from build123d import *

# Parameters (mm, degrees)
BOSS_EXTRU_1_DEPTH                                  = 40
ESQUISSE1_4_W                                       = 16
ESQUISSE1_4_H                                       = 96
BOSS_EXTRUDE1_DEPTH                                 = 30
ESQUISSE3_R                                         = 14
ENL_V_MAT_EXTRU_2_DEPTH                             = 40
CONG_1_R                                            = 6
CBORE_FOR_M8_HEX_SOCKET_HEAD_CAP_SCREW2_D           = 9
CBORE_FOR_M8_HEX_SOCKET_HEAD_CAP_SCREW2_CBORE_D     = 15
CBORE_FOR_M8_HEX_SOCKET_HEAD_CAP_SCREW2_CBORE_DEPTH = 8.6
SKETCH7_R                                           = 24.5
CUT_EXTRUDE2_DEPTH                                  = 9
M5_TAPPED_HOLE2_D                                   = 4.2
M5_TAPPED_HOLE2_DEPTH                               = 14
M5_TAPPED_HOLE2_TIP                                 = 1.2618073
SKETCH12_R                                          = 9
CUT_EXTRUDE3_DEPTH                                  = 151
TAP_DRILL_FOR_M6_TAP2_AT_2_COUNT                    = 2
TAP_DRILL_FOR_M6_TAP2_AT_2_PITCH                    = 24
TAP_DRILL_FOR_M6_TAP2_AT_3_COUNT                    = 2
TAP_DRILL_FOR_M6_TAP2_AT_3_PITCH                    = 110
TAP_DRILL_FOR_M6_TAP2_AT_4_COUNT                    = 2
TAP_DRILL_FOR_M6_TAP2_AT_4_PITCH                    = 112.58774356
FILLET2_R                                           = 5
FILLET3_R                                           = 6
FILLET4_R                                           = 2
TAP_DRILL_FOR_M6_TAP1_D                             = 5
TAP_DRILL_FOR_M6_TAP1_DEPTH                         = 23
TAP_DRILL_FOR_M6_TAP1_TIP                           = 1.502151548
FILLET1_R                                           = 1
CHAMFER1_SIZE                                       = 0.5


with BuildPart() as part:
    # Esquisse1 → Boss.-Extru.1 (new body)
    with BuildSketch(Plane.XY):
        Polygon((58.5, -48), (42.5, -48), (42.5, 48), (58.5, 48), (58.5, 105), (-58.5, 105), (-58.5, 48), (-42.5, 48), (-42.5, -48), (-58.5, -48), (-58.5, -85), (-10, -85), (-10, 55), (10, 55), (10, -85), (58.5, -85), align=None)
    extrude(amount=BOSS_EXTRU_1_DEPTH)

    # Esquisse1_4 → Boss-Extrude1 (add)
    with BuildSketch(Plane.XY):
        with Locations((-50.5, 0)):
            Rectangle(ESQUISSE1_4_W, ESQUISSE1_4_H)
        with Locations((50.5, 0)):
            Rectangle(ESQUISSE1_4_W, ESQUISSE1_4_H)
    extrude(amount=BOSS_EXTRUDE1_DEPTH)

    # Esquisse3 → Enl_v. mat.-Extru.2 (cut)
    with BuildSketch(Plane(origin=(0, 105, 0), x_dir=(1, 0, 0), z_dir=(0, 1, 0))):
        with Locations((0, -20)):
            Circle(ESQUISSE3_R)
    extrude(amount=-ENL_V_MAT_EXTRU_2_DEPTH, mode=Mode.SUBTRACT)

    # Cong_1
    cong_1_edges = [part.edges().sort_by_distance(p)[0] for p in [
        (10, 55, 20),
        (-10, 55, 20),
    ]]
    fillet(cong_1_edges, radius=CONG_1_R)

    # CBORE for M8 Hex Socket Head Cap Screw2 (through all)
    with Locations(Plane.XY.offset(40)):
        with Locations((-22.5, 73.5), (22.5, 73.5), (22.5, 16.5), (-22.5, 16.5), (-22.5, -16.5), (22.5, -16.5), (22.5, -73.5), (-22.5, -73.5)):
            CounterBoreHole(CBORE_FOR_M8_HEX_SOCKET_HEAD_CAP_SCREW2_D / 2, CBORE_FOR_M8_HEX_SOCKET_HEAD_CAP_SCREW2_CBORE_D / 2, CBORE_FOR_M8_HEX_SOCKET_HEAD_CAP_SCREW2_CBORE_DEPTH)

    # Sketch7 → Cut-Extrude2 (cut)
    with BuildSketch(Plane(origin=(0, 105, 0), x_dir=(1, 0, 0), z_dir=(0, 1, 0))):
        with Locations((0, -20)):
            Circle(SKETCH7_R)
    extrude(amount=-CUT_EXTRUDE2_DEPTH, mode=Mode.SUBTRACT)

    # M5 Tapped Hole2
    with Locations(Plane(origin=(0, 96, 0), x_dir=(1, 0, 0), z_dir=(0, 1, 0))):
        with Locations((-13.435028843, -6.564971157), (-19, -20), (13.435028843, -6.564971157), (19, -20), (13.435028843, -33.435028843), (-13.435028843, -33.435028843)):
            Hole(M5_TAPPED_HOLE2_D / 2, depth=M5_TAPPED_HOLE2_DEPTH)
            with Locations((0, 0, -(M5_TAPPED_HOLE2_DEPTH + M5_TAPPED_HOLE2_TIP / 2))):  # 118° drill point
                Cone(0, M5_TAPPED_HOLE2_D / 2, M5_TAPPED_HOLE2_TIP, mode=Mode.SUBTRACT)

    # Sketch12 → Cut-Extrude3 (cut, through all)
    with BuildSketch(Plane(origin=(0, 65, 0), x_dir=(1, 0, 0), z_dir=(0, 1, 0))):
        with Locations((0, -20)):
            Circle(SKETCH12_R)
    extrude(amount=-CUT_EXTRUDE3_DEPTH, mode=Mode.SUBTRACT)

    # Sketch14 → Tap Drill for M6 Tap2 (revolve, cut)
    with BuildSketch(Plane(origin=(58.5, 55, 8), x_dir=(0, 0, -1), z_dir=(0, 1, 0))):
        Polygon((0, 0), (0, 11.502151548), (2.5, 10), (2.5, 0), align=None)
    tap_drill_for_m6_tap2 = revolve(axis=Axis((64.85, 55, 8), (-1, 0, 0)), mode=Mode.SUBTRACT)

    # Tap Drill for M6 Tap2 at 2: Tap Drill for M6 Tap2 ×2
    with Locations(*[(0, 0, i * TAP_DRILL_FOR_M6_TAP2_AT_2_PITCH) for i in range(1, TAP_DRILL_FOR_M6_TAP2_AT_2_COUNT)]):
        add(tap_drill_for_m6_tap2, mode=Mode.SUBTRACT)

    # Tap Drill for M6 Tap2 at 3: Tap Drill for M6 Tap2 ×2
    with Locations(*[(0, -i * TAP_DRILL_FOR_M6_TAP2_AT_3_PITCH, 0) for i in range(1, TAP_DRILL_FOR_M6_TAP2_AT_3_COUNT)]):
        add(tap_drill_for_m6_tap2, mode=Mode.SUBTRACT)

    # Tap Drill for M6 Tap2 at 4: Tap Drill for M6 Tap2 ×2
    with Locations(*[Vector(0, -0.977015761, 0.213167075) * (i * TAP_DRILL_FOR_M6_TAP2_AT_4_PITCH) for i in range(1, TAP_DRILL_FOR_M6_TAP2_AT_4_COUNT)]):
        add(tap_drill_for_m6_tap2, mode=Mode.SUBTRACT)

    # Mirror1: Tap Drill for M6 Tap2 across plane
    add(tap_drill_for_m6_tap2.mirror(Plane(origin=(0, 0, 0), x_dir=(0, 0, 1), z_dir=(1, 0, 0))), mode=Mode.SUBTRACT)

    # Mirror1 copy 1 sketch → Mirror1 copy 1 (revolve, cut)
    with BuildSketch(Plane(origin=(-58.5, 55, 32), x_dir=(0, 0, -1), z_dir=(0, 1, 0))):
        Polygon((0, 0), (0, -11.502151548), (2.5, -10), (2.5, 0), align=None)
    revolve(axis=Axis((-64.85, 55, 32), (-1, 0, 0)), mode=Mode.SUBTRACT)

    # Mirror1 copy 2 sketch → Mirror1 copy 2 (revolve, cut)
    with BuildSketch(Plane(origin=(-58.5, -55, 8), x_dir=(0, 0, -1), z_dir=(0, 1, 0))):
        Polygon((0, 0), (0, -11.502151548), (2.5, -10), (2.5, 0), align=None)
    revolve(axis=Axis((-64.85, -55, 8), (-1, 0, 0)), mode=Mode.SUBTRACT)

    # Mirror1 copy 3 sketch → Mirror1 copy 3 (revolve, cut)
    with BuildSketch(Plane(origin=(-58.5, -55, 32), x_dir=(0, 0, -1), z_dir=(0, 1, 0))):
        Polygon((0, 0), (0, -11.502151548), (2.5, -10), (2.5, 0), align=None)
    revolve(axis=Axis((-64.85, -55, 32), (-1, 0, 0)), mode=Mode.SUBTRACT)

    # Fillet2
    fillet2_edges = [part.edges().sort_by_distance(p)[0] for p in [
        (10, -85, 20),
        (-10, -85, 20),
    ]]
    fillet(fillet2_edges, radius=FILLET2_R)

    # Fillet3
    fillet3_edges = [part.edges().sort_by_distance(p)[0] for p in [
        (-42.5, -48, 35),
        (-42.5, 48, 35),
        (42.5, 48, 35),
        (42.5, -48, 35),
    ]]
    fillet(fillet3_edges, radius=FILLET3_R)

    # Fillet4
    fillet4_edges = [part.edges().sort_by_distance(p)[0] for p in [
        (58.5, -48, 35),
        (-58.5, -48, 35),
        (-58.5, 48, 35),
        (58.5, 48, 35),
    ]]
    fillet(fillet4_edges, radius=FILLET4_R)

    # Tap Drill for M6 Tap1
    with Locations(Plane(origin=(0, 105, 0), x_dir=(1, 0, 0), z_dir=(0, 1, 0))):
        with Locations((-51, -30), (-51, -10), (51, -10), (51, -30)):
            Hole(TAP_DRILL_FOR_M6_TAP1_D / 2, depth=TAP_DRILL_FOR_M6_TAP1_DEPTH)
            with Locations((0, 0, -(TAP_DRILL_FOR_M6_TAP1_DEPTH + TAP_DRILL_FOR_M6_TAP1_TIP / 2))):  # 118° drill point
                Cone(0, TAP_DRILL_FOR_M6_TAP1_D / 2, TAP_DRILL_FOR_M6_TAP1_TIP, mode=Mode.SUBTRACT)

    # Fillet1
    fillet1_edges = [part.edges().sort_by_distance(p)[0] for p in [
        (-14.150971698, 100.5, 0),
        (14.150971698, 100.5, 0),
        (14.150971698, 100.5, 40),
        (-14.150971698, 100.5, 40),
    ]]
    fillet(fillet1_edges, radius=FILLET1_R)

    # Chamfer1
    chamfer1_edges = [part.edges().sort_by_distance(p)[0] for p in [
        (15, -73.5, 40),
        (15, -16.5, 40),
        (-30, -16.5, 40),
        (-30, 16.5, 40),
        (15, 16.5, 40),
        (15, 73.5, 40),
        (-30, 73.5, 40),
        (-14, 96, 20),
        (37.753675676, 105, 40),
        (37.753675676, 105, 0),
        (10, -15.5, 40),
        (-36.75, -85, 40),
        (-10, -15.5, 40),
        (-11.464466094, -83.535533906, 40),
        (11.464466094, -83.535533906, 40),
        (-42.5, 0, 40),
        (42.5, 0, 40),
        (-44.257359313, 46.242640687, 40),
        (-44.257359313, -46.242640687, 40),
        (44.257359313, -46.242640687, 40),
        (44.257359313, 46.242640687, 40),
        (52.5, -48, 40),
        (58.5, 77.5, 40),
        (52.5, 48, 40),
        (-58.5, 77.5, 40),
        (-52.5, 48, 40),
        (-52.5, -48, 40),
        (-57.914213562, 48.585786438, 40),
        (-57.914213562, -48.585786438, 40),
        (57.914213562, 48.585786438, 40),
        (57.914213562, -48.585786438, 40),
        (-58.5, 105, 20),
        (58.5, 105, 20),
        (53.5, 105, 30),
        (53.5, 105, 10),
        (-48.5, 105, 10),
        (-48.5, 105, 30),
        (24.5, 105, 20),
        (16.073248028, 105, 0.642997226),
        (16.073248028, 105, 39.357002774),
        (-37.753675676, 105, 40),
        (-24.5, 105, 20),
        (-37.753675676, 105, 0),
        (-16.073248028, 105, 0.642997226),
        (-16.073248028, 105, 39.357002774),
        (-58.5, -67.5, 40),
        (36.75, -85, 40),
        (58.5, -67.5, 40),
        (0, 55, 40),
        (8.242640687, 53.242640687, 40),
        (-8.242640687, 53.242640687, 40),
        (-30, -73.5, 40),
    ]]
    chamfer(chamfer1_edges, length=CHAMFER1_SIZE)


solid = part.part
Source: CAD feature listing. Evaluate the final solid. Frame: model axes, mm. A direction names the side the tool comes from. Coordinates: 2 decimals unless noted, no trailing zeros. Order: outer loops, then holes, each group sorted by start corner. A loop starts at its lowest first (then second) coordinate and runs counter-clockwise, first axis right, second up.
Item 1: Cut plane B-B (y = 1.5). Return loops of the section in (x, z), plus the area to 3 significant figures.
Output values:
outline: (-58.5, 0) - (-10, 0) - (-10, 39.5) - (-10.5, 40) - (-42, 40) - (-42.5, 39.5) - (-42.5, 30) - (-58.5, 30) - close; (10, 0) - (58.5, 0) - (58.5, 30) - (42.5, 30) - (42.5, 39.5) - (42, 40) - (10.5, 40) - (10, 39.5) - close
area: 3,560 mm2
Item 2: Pull-direction query (Z, two-part tool) for faces 6 (the face through (-52.34, 93.09, 27.89)), 7 (the face through (-53.57, 57.44, 8.54)), 8 (the face through (10, -15, 19)), 9 (the face through (26, -20, 31.4)); classes: pulls with the +Z half, pulls with the -Z half, needs draft (parallel to the pull), parting line crosses it, or undercut.
Output values:
face 6: undercut
face 7: undercut
face 8: needs draft
face 9: pulls with the +Z half
Item 3: Cut plane A-A (y = -73.5). Count the separate pieces of the cut face and the enclosed holes in it, plus the area to 3 significant figures.
Output values:
separate pieces: 4
enclosed holes: 0
area: 3,060 mm2
Item 4: First-contact query: P1, Ø12, axis at x = -7, y = 8.5, coming from the +Z side; P2, Ø7.5, axis at x = -22.5, y = -14.5, coming from the +Z side; P3, Ø3, axis at y = 17, z = 36.5, coming from the -X side; P4, Ø5.5, axis at x = 22.5, y = -16.5, coming from the -Z side. Flat tips, straight axial feed; report the tip coordinate or a pass-through.
Output values:
P1: stops at z = 40
P2: stops at z = 31.4
P3: stops at x = -42.5
P4: passes through
Item 5: Set-up query: faces 1 (the face through (44.21, -46.39, 39.64)), 2 (the face through (9.41, 51.595, 20.026)), 3 (the face through (16.548, 68.936, 35.507)), 4 (the face through (-14.4, 88.9, 35.3)), 5 (the face through (53.57, -52.56, 8.54)). Return all of +Z, -Z, +X, -X, +Y, -Y with unobstructed straight access to the full face (end or side cutting, diameter ignored); none if empty.
Output values:
face 1: +Z, +X
face 2: +Z, -Z, -Y
face 3: +Z
face 4: +Y
face 5: +X
Item 6: Material intervals for line 1 (Z direction, x = 53.25, y = 55); line 2 (Z direction, x = -51, y = 99.5); line 3 (Y direction, x = 55.75, z = 8), sorted ascending.
Output values:
line 1: z = 0 to 5.5, 10.5 to 29.5, 34.5 to 40
line 2: z = 0 to 7.5, 12.5 to 27.5, 32.5 to 40
line 3: y = -85 to -57.5, -52.5 to 52.5, 57.5 to 105
